Source: three-view drawing plus pictorial views. Frame: mm from the lowest corner of the part. A direction names the side the tool comes from. Coordinates: 2 decimals unless noted, no trailing zeros. Write each loop counter-clockwise with the first axis right and the second up, starting at its lowest first coordinate (ties: lowest second). Pieces come first, ordered by that corner, then holes. Notation, with made-up numbers: (12, 59.25) - (18, 59.25) arc R20 cw to (18, 75.25) - close; hole circle Ø7 at (68, -1.5). An arc over 180 degrees is marked (long way). Answer as a JSON object with one key per item and string values. Group by question number.
Item 1: Line query: line 1 along Z through (x, y) = (2.5, 7.5); line 2 along X through (y, z) = (6, 1); line 3 along X through (y, z) = (3.75, 1). Output: solid intervals per line, ascending. Write a range as from..to.
Item 2: Set-up query: the marked faces 1, 2, 3, 4 and 5. Return all of +Z, -Z, +X, -X, +Y, -Y with unobstructed straight access to the full face (end or side cutting, diameter ignored); none if empty.
Item 3: Section A-A on z = 1. Return loops of the section in (x, y).
Item 4: Section C-C on y = 1. Return loops of the section in (x, z).
Item 5: Section D-D on x = 3.3. Return loops of the section in (y, z), and give its area (3 significant figures).
Item 6: Section B-B on x = 2.5. Return loops of the section in (y, z).
Item 7: First-contact query: pin 1 Ø0.8 at (x, y) = (4, 6.5) entering from -Z; pin 2 Ø0.5 at (y, z) = (7, 1) entering from +X; pin 3 Ø0.6 at (y, z) = (6.5, 0.5) entering from -X. Flat tips, straight axial feed; report the tip coordinate or a pass-through.
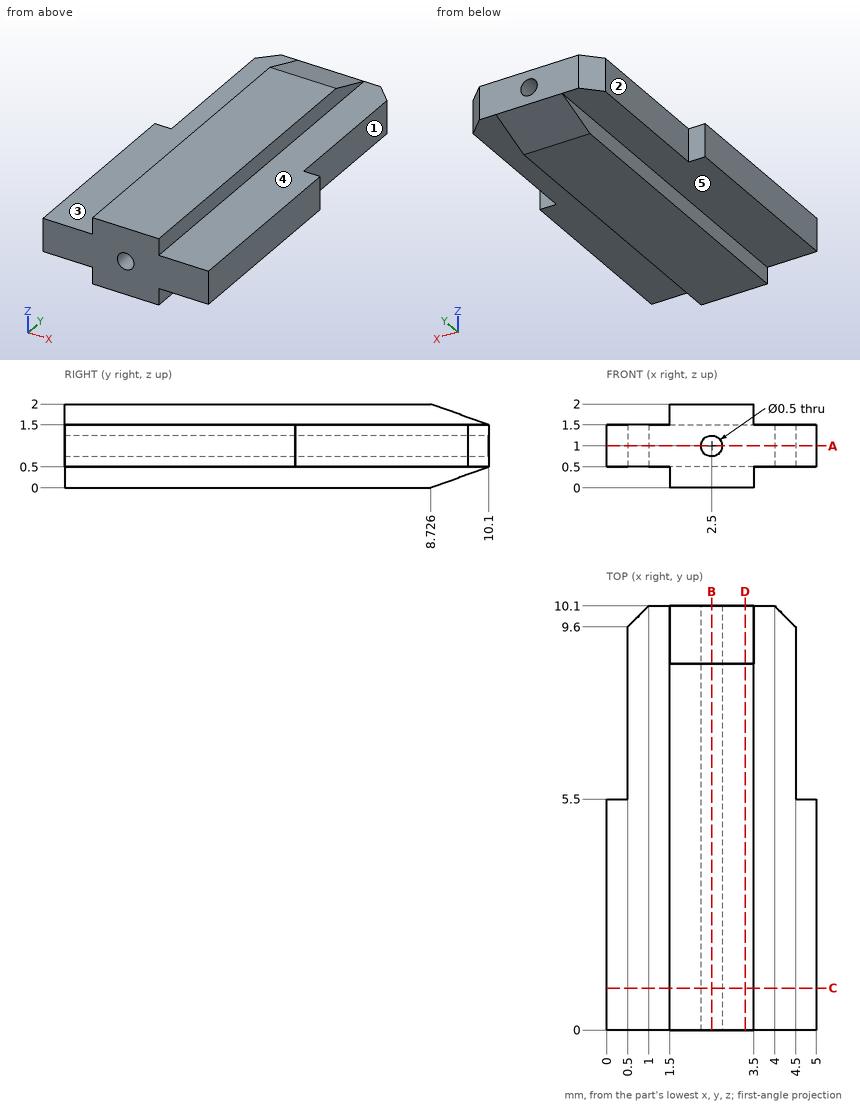
Checks:
{
 "1": {"line 1": "0..0.75, 1.25..2", "line 2": "0.5..2.25, 2.75..4.5", "line 3": "0..2.25, 2.75..5"},
 "2": {"face 1": "+Z, -Z, +X, +Y", "face 2": "+Z, -Z, -X, +Y", "face 3": "+Z, -X, +Y, -Y", "face 4": "+Z, +X, +Y, -Y", "face 5": "-Z, -X, +Y, -Y"},
 "3": {"outline": "(0, 0) - (2.25, 0) - (2.25, 10.1) - (1, 10.1) - (0.5, 9.6) - (0.5, 5.5) - (0, 5.5) - close; (2.75, 0) - (5, 0) - (5, 5.5) - (4.5, 5.5) - (4.5, 9.6) - (4, 10.1) - (2.75, 10.1) - close"},
 "4": {"outline": "(0, 0.5) - (1.5, 0.5) - (1.5, 0) - (3.5, 0) - (3.5, 0.5) - (5, 0.5) - (5, 1.5) - (3.5, 1.5) - (3.5, 2) - (1.5, 2) - (1.5, 1.5) - (0, 1.5) - close; hole circle Ø0.5 at (2.5, 1)"},
 "5": {"outline": "(0, 0) - (8.73, 0) - (10.1, 0.5) - (10.1, 1.5) - (8.73, 2) - (0, 2) - close", "area": "19.5 mm^2"},
 "6": {"outline": "(0, 0) - (8.73, 0) - (10.1, 0.5) - (10.1, 0.75) - (0, 0.75) - close; (0, 1.25) - (10.1, 1.25) - (10.1, 1.5) - (8.73, 2) - (0, 2) - close"},
 "7": {"pin 1": "z = 0.5", "pin 2": "x = 4.5", "pin 3": "x = 0.5"}
}
